```python
from build123d import *

# Parameters (mm, degrees)
F0_R          = 14.2875
F0_R_2        = 9.779
F1_DEPTH      = 12.7
F3_DEPTH      = 1.905
F3_DEPTH_BACK = 1.905
F5_DEPTH      = 12.7


with BuildPart() as f1:
    # F0 (on Top) → F1 (new body)
    with BuildSketch(Plane.XY):
        Circle(F0_R)
        Circle(F0_R_2, mode=Mode.SUBTRACT)
    extrude(amount=F1_DEPTH)

    # F2 (on Front) → F3 (join, two sides)
    with BuildSketch(Plane.XZ) as f3_sk:
        with BuildLine():
            Line((13.3136538789, 12.7235082909), (13.3136538789, 6.35))
            Line((13.3136538789, 6.35), (29.845, 6.35))
            ThreePointArc((29.845, 6.35), (30.994771982, 10.18931491), (34.0655694999, 12.7646823))
            ThreePointArc((34.0655694999, 12.7646823), (24.1589088565, 11.7366418782), (14.2480619252, 12.7235082909))
            Line((14.2480619252, 12.7235082909), (13.3136538789, 12.7235082909))
        make_face()
        with BuildLine():
            Line((29.845, 6.35), (13.3136538789, 6.35))
            Line((13.3136538789, 6.35), (13.3136538789, 0))
            Line((13.3136538789, 0), (14.5748257637, 0))
            ThreePointArc((14.5748257637, 0), (24.1986734185, 0.7965285613), (33.8260559146, 0.0439279316))
            ThreePointArc((33.8260559146, 0.0439279316), (30.9235300544, 2.6212149725), (29.845, 6.35))
        make_face()
        with BuildLine():
            ThreePointArc((34.0655694999, 12.7646823), (30.994771982, 10.18931491), (29.845, 6.35))
            ThreePointArc((29.845, 6.35), (30.9235300544, 2.6212149725), (33.8260559146, 0.0439279316))
            ThreePointArc((33.8260559146, 0.0439279316), (35.5736615146, -0.2615447543), (37.311506327, -0.6183840779))
            ThreePointArc((37.311506327, -0.6183840779), (41.9365422105, 1.5841368407), (43.815, 6.35))
            ThreePointArc((43.815, 6.35), (41.6376310588, 11.4172387552), (36.4629860837, 13.3253513019))
            ThreePointArc((36.4629860837, 13.3253513019), (35.2677832143, 13.0300276397), (34.0655694999, 12.7646823))
        make_face()
        with BuildLine():
            ThreePointArc((39.497, 6.35), (36.83, 3.683), (34.163, 6.35))
            ThreePointArc((34.163, 6.35), (36.83, 9.017), (39.497, 6.35))
        make_face(mode=Mode.SUBTRACT)
        with BuildLine():
            ThreePointArc((36.4629860837, 13.3253513019), (35.2393795344, 13.1514815691), (34.0655694999, 12.7646823))
            ThreePointArc((34.0655694999, 12.7646823), (35.2677832143, 13.0300276397), (36.4629860837, 13.3253513019))
        make_face()
        with BuildLine():
            ThreePointArc((37.311506327, -0.6183840779), (35.5736615146, -0.2615447543), (33.8260559146, 0.0439279316))
            ThreePointArc((33.8260559146, 0.0439279316), (35.5260301534, -0.5122071988), (37.311506327, -0.6183840779))
        make_face()
    extrude(amount=F3_DEPTH)
    extrude(f3_sk.sketch, amount=-F3_DEPTH_BACK)

    # F4 (on face) → F5 (join, through all)
    with BuildSketch(Plane.XY.offset(12.7)):
        with BuildLine():
            ThreePointArc((17.3360537738, 1.9065266242), (15.2188372166, 2.8229826148), (13.5784069673, 4.4451682175))
            ThreePointArc((13.5784069673, 4.4451682175), (13.9272019714, 3.188369724), (14.1599304818, 1.905))
            Line((14.1599304818, 1.905), (13.4946856848, 1.905))
            Line((13.4946856848, 1.905), (13.4318988812, 0))
            Line((13.4318988812, 0), (17.3360537738, 0))
            Line((17.3360537738, 0), (17.3360537738, 1.9065266242))
        make_face()
        with BuildLine():
            ThreePointArc((14.1599304818, -1.905), (13.8146153266, -3.6454162489), (13.2562405183, -5.3296100767))
            ThreePointArc((13.2562405183, -5.3296100767), (15.0043175715, -3.2852044457), (17.3360537738, -1.9441697514))
            Line((17.3360537738, -1.9441697514), (17.3360537738, 0))
            Line((17.3360537738, 0), (13.4318988812, 0))
            Line((13.4318988812, 0), (13.3691120776, -1.905))
            Line((13.3691120776, -1.905), (14.1599304818, -1.905))
        make_face()
    extrude(amount=-F5_DEPTH)


solid = f1.part
```
The model under review builds one solid part; all positions refer to its coordinate system, in mm. A direction names the side the tool comes from. Give positions to 0.01 mm unless a question says otherwise; leave off trailing zeros. Write each loop counter-clockwise with the first axis right and the second up, starting at its lowest first coordinate (ties: lowest second). Pieces come first, ordered by that corner, then holes.
(1) The part is to be moulded in two halves that separate along X. For faces 4 (the flat face through (17.336, 0, 12.5)), 5 (the flat face through (1, 10, 0)), 6 (the cylindrical face through (14.975, -3.309, 6.439)), say which applies: released by +X, released by -X, zero draft, split by the parting line, or undercut.
(2) For P1, Ø1, axis at x = 16, z = 3.5, coming from the -Y side; P2, Ø6, axis at y = -7.5, z = 7.5, coming from the -X side; P3, Ø7, axis at x = 36, z = 9.5, coming from the +Y side (3 decimals), all flat-tipped, find the tip position at first contact; note any pin that passes through.
(3) Tool access review of faces 1 (the flat face through (30, -1.905, 6)), 2 (the cylindrical face through (-14.25, 1.03, 6.26)), 3 (the flat face through (30, 1.905, 6)): name each direction out of +Z, -Z, +X, -X, +Y, -Y from which nothing blocks a thin tool from reaching the whole face with its end or side.
(4) Consider section A-A, the plane x = 0. Give the boundary of the cut face in (y, z).
(5) To check wall thickness, follow L1, parallel to Y at x = 0, z = 9.5; L2, parallel to Z at x = 36.83, y = -0.8 (3 decimals); L3, parallel to X at y = 0.5, z = 8.5. State the ranges of each line that lie inside material, in increasing order.
(6) Consider section B-B, the plane y = -4.5. Give the boundary of the cut face in (x, z).
(7) Consider section C-C, the plane z = 5.75. Give the number of separate pieces and of enclosed holes in the cut face, and give its area (3 significant figures).
(8) Consider section D-D, the plane x = 31. Give the boundary of the cut face in (y, z) (3 decimals).
Returned:
1. face 4: undercut
1. face 5: zero draft
1. face 6: released by +X
2. P1: stops at y = -2.91
2. P2: stops at x = -13.56
2. P3: stops at y = 1.905
3. face 1: +Z, -Z, +X, -Y
3. face 2: +Z, -Z
3. face 3: +Z, -Z, +X, +Y
4. outline: (-14.29, 0) - (-9.78, 0) - (-9.78, 12.7) - (-14.29, 12.7) - close; (9.78, 0) - (14.29, 0) - (14.29, 12.7) - (9.78, 12.7) - close
5. L1: y = -14.29 to -9.78, 9.78 to 14.29
5. L2: z = -0.635 to 3.683, 9.017 to 13.335
5. L3: x = -14.28 to -9.77, 9.77 to 35.25, 38.41 to 43.48
6. outline: (-13.56, 0) - (-8.68, 0) - (-8.68, 12.7) - (-13.56, 12.7) - close; (8.68, 0) - (13.82, 0) - (13.82, 12.7) - (8.68, 12.7) - close
7. separate pieces: 2
7. enclosed holes: 1
7. area: 440 mm2
8. outline: (-1.905, 0.427) - (1.905, 0.427) - (1.905, 12.229) - (-1.905, 12.229) - close
